from build123d import *

# Parameters (mm, degrees)
SKETCH1_W           = 43.55
SKETCH1_H           = 11
SKETCH1_W_2         = 21.55
SKETCH1_H_2         = 7
BOSS_EXTRUDE1_DEPTH = 3
SKETCH1_2_W         = 43.55
SKETCH1_2_H         = 11
SKETCH1_2_W_2       = 21.55
SKETCH1_2_H_2       = 7
BOSS_EXTRUDE2_DEPTH = 3


with BuildPart() as part:
    # Sketch1 → Boss-Extrude1 (new body)
    with BuildSketch(Plane(origin=(0, 0, 0), x_dir=(1, 0, 0), z_dir=(0, 1, 0))):
        with Locations((21.775, -5.5)):
            Rectangle(SKETCH1_W, SKETCH1_H)
        with Locations((12.775, -5.5)):
            Rectangle(SKETCH1_W_2, SKETCH1_H_2, mode=Mode.SUBTRACT)
    extrude(amount=BOSS_EXTRUDE1_DEPTH)

    # Sketch1_2 → Boss-Extrude2 (add)
    with BuildSketch(Plane(origin=(0, 0, 0), x_dir=(1, 0, 0), z_dir=(0, 1, 0))):
        with Locations((21.775, -5.5)):
            Rectangle(SKETCH1_2_W, SKETCH1_2_H)
        with Locations((12.775, -5.5)):
            Rectangle(SKETCH1_2_W_2, SKETCH1_2_H_2, mode=Mode.SUBTRACT)
        with Locations((12.775, -5.5)):
            Rectangle(SKETCH1_2_W_2, SKETCH1_2_H_2)
    extrude(amount=-BOSS_EXTRUDE2_DEPTH)


solid = part.part
Design review of the part built by this model. Coordinates are the model's own, in mm. A direction names the side the tool comes from. Round coordinates to 2 decimals unless told otherwise and drop trailing zeros. Write each loop counter-clockwise with the first axis right and the second up, starting at its lowest first coordinate (ties: lowest second). Pieces come first, ordered by that corner, then holes. Notation, with made-up numbers: (65.5, 2.25) - (80.5, 2.25) arc R21 cw to (80.5, 7.25) - close; hole circle Ø11 at (8, -16). An arc over 180 degrees is marked (long way). Use a Markdown table: item, result. Add a question column.
1. We need section B-B (x = 3). State the section outline as (y, z) points.
2. We need section A-A (y = 1.05). State the section outline as (x, z) points, then the cut area to 3 significant figures.
3. Wall thickness on probe 1 along Z at (x, y) = (6, 1.7); probe 2 along X at (y, z) = (0.45, 7.25); probe 3 along Y at (x, z) = (2.5, 6): over which ranges is each line inside the solid? List them lowest first.
4. Mouldability with a two-part tool opening along X and no side actions: class faces 3 (the face through (26, 3, 5)), 4 (the face through (13, 1, 2)), 5 (the face through (0, 0, 6)) as +X half, -X half, draft (parallel to the pull), parting line (faces both ways), or undercut.
5. For faces 1 (the face through (21, 0, 11)), 2 (the face through (2, 1, 6)), list the 3-axis set-ups (+Z, -Z, +X, -X, +Y, -Y) from which the entire face can be reached by the end or side of a thin tool; tool diameter is ignored.
6. Clearance check with a flat-ended pin moving along its axis: pin 1 (1 mm diameter, centred on x = 16.5, z = 6, fed in from +Y). State where the tip first meets the part, or that it passes through.
7. We need section C-C (z = 8). State the section outline as (x, y) points, then the cut area to 3 significant figures.
Output:
| question | item | result |
|---|---|---|
| 1 | outline | (-3, 0) - (3, 0) - (3, 2) - (0, 2) - (0, 9) - (3, 9) - (3, 11) - (-3, 11) - close |
| 2 | outline | (0, 0) - (43.55, 0) - (43.55, 11) - (0, 11) - close; hole (2, 2) - (23.55, 2) - (23.55, 9) - (2, 9) - close |
| 2 | area | 328 mm2 |
| 3 | probe 1 | z = 0 to 2, 9 to 11 |
| 3 | probe 2 | x = 0 to 2, 23.55 to 43.55 |
| 3 | probe 3 | y = -3 to 0 |
| 4 | face 3 | draft |
| 4 | face 4 | undercut |
| 4 | face 5 | -X half |
| 5 | face 1 | +Z, +X, -X, +Y, -Y |
| 5 | face 2 | +Y |
| 6 | pin 1 | stops at y = 0 |
| 7 | outline | (0, -3) - (43.55, -3) - (43.55, 3) - (23.55, 3) - (23.55, 0) - (2, 0) - (2, 3) - (0, 3) - close |
| 7 | area | 197 mm2 |
